from build123d import *

# Parameters (mm, degrees)
SKETCH1_R           = 6.35
BOSS_EXTRUDE1_DEPTH = 38.1
BOSS_EXTRUDE2_DEPTH = 12.7
SKETCH3_R           = 6.35
BOSS_EXTRUDE3_DEPTH = 25.4


with BuildPart() as part:
    # Sketch1 → Boss-Extrude1 (new body)
    with BuildSketch(Plane.XY):
        with Locations(Location((0, 0, 0), (0, 0, 180))):
            Circle(SKETCH1_R)
    extrude(amount=BOSS_EXTRUDE1_DEPTH)

    # Sketch2 → Boss-Extrude2 (add)
    with BuildSketch(Plane.XY.offset(38.1)):
        with BuildLine():
            Line((-4.445, -4.534807052), (4.445, -4.534807052))
            Line((4.445, -4.534807052), (4.445, 4.534807052))
            ThreePointArc((4.445, 4.534807052), (-4.534807052, 4.445), (-4.445, -4.534807052))
        make_face()
    extrude(amount=BOSS_EXTRUDE2_DEPTH)

    # Sketch3 → Boss-Extrude3 (add)
    with BuildSketch(Plane.XY.offset(50.8)):
        Circle(SKETCH3_R)
    extrude(amount=BOSS_EXTRUDE3_DEPTH)


solid = part.part
For this review, take the finished solid that the model builds, in its own axes (mm). A direction names the side the tool comes from. Round coordinates to 2 decimals unless told otherwise and drop trailing zeros. Order: outer loops, then holes, each group sorted by start corner. A loop starts at its lowest first (then second) coordinate and runs counter-clockwise, first axis right, second up. Notation, with made-up numbers: (-2.75, 46) -> (53.25, 46) arc R19 ccw to (53.25, 52) -> close; hole circle Ø8 at (-2.75, 77). An arc over 180 degrees is marked (long way). Put each result on its own line as item: value.
Q1. For probe 1 along Y at (x, z) = (0.25, 39); probe 2 along X at (y, z) = (-2, 32); probe 3 along Y at (x, z) = (-4, 4.5), list the stretches that pass through material, from the lowest coordinate up. Write a range as [from, to].
Check result:
probe 1: [-4.53, 6.35]
probe 2: [-6.03, 6.03]
probe 3: [-4.93, 4.93]
Q2. Add section C-C on x = 0. Write out the cut boundary in (y, z).
Check result:
outline: (-6.35, 0) -> (6.35, 0) -> (6.35, 76.2) -> (-6.35, 76.2) -> (-6.35, 50.8) -> (-4.53, 50.8) -> (-4.53, 38.1) -> (-6.35, 38.1) -> close
Q3. Insertion check: pin 1 Ø4 at (x, z) = (2.5, 68) entering from +Y; pin 2 Ø2 at (x, z) = (2.5, 31) entering from +Y; pin 3 Ø2.5 at (x, z) = (-1, 47) entering from -Y. Each pin has a flat end and moves straight along its axis. Give the tip position at first contact, or say it passes through.
Check result:
pin 1: y = 6.33
pin 2: y = 6.17
pin 3: y = -4.53
Q4. Machinability: for faces 1 (the flat face through (0, -5, 50.8)), 2 (the flat face through (4.445, 0, 44)), which of the approach directions +Z, -Z, +X, -X, +Y, -Y give a long, thin tool a straight path to every point of the face, cutting with its end or side? Answer none if there is none.
Check result:
face 1: +X, -X, -Y
face 2: +X, +Y, -Y
Q5. Mouldability with a two-part tool opening along Z and no side actions: class faces 3 (the flat face through (0, 0, 0)), 4 (the flat face through (5, 0, 50.8)), 5 (the flat face through (0, 0, 76.2)) as pulls with the +Z half, pulls with the -Z half, needs draft (parallel to the pull), parting line crosses it, or undercut.
Check result:
face 3: pulls with the -Z half
face 4: undercut
face 5: pulls with the +Z half
Q6. Add section B-B on y = 0. Write out the cut boundary in (x, z) (3 decimals), plus the area to 3 significant figures.
Check result:
outline: (-6.35, 0) -> (6.35, 0) -> (6.35, 38.1) -> (4.445, 38.1) -> (4.445, 50.8) -> (6.35, 50.8) -> (6.35, 76.2) -> (-6.35, 76.2) -> close
area: 944 mm2
Q7. Add section A-A on x = 5.25. Write out the cut boundary in (y, z), plus the area to 3 significant figures.
Check result:
outline: (-3.57, 0) -> (3.57, 0) -> (3.57, 38.1) -> (-3.57, 38.1) -> close; (-3.57, 50.8) -> (3.57, 50.8) -> (3.57, 76.2) -> (-3.57, 76.2) -> close
area: 454 mm2
Q8. Add section D-D on z = 69.5. Write out the cut boundary in (x, y).
Check result:
outline: circle Ø12.7 at (0, 0)
